Input: part model. Units: mm. Frame: model coordinates. A direction names the side the tool comes from. Coordinates: 2 decimals unless noted, no trailing zeros. Write each loop counter-clockwise with the first axis right and the second up, starting at its lowest first coordinate (ties: lowest second). Pieces come first, ordered by that corner, then holes. Notation, with made-up numbers: (7.5, 42.5) -> (56.5, 42.5) arc R25 cw to (56.5, 65.5) -> close; hole circle Ø9 at (-21, -36.75). An arc over 180 degrees is marked (long way). One line per question, with ' | ' between items. Start each with the question number.
```python
from build123d import *

# Parameters (mm, degrees)
SKETCH1_W           = 25.4
SKETCH1_H           = 24.3078
BOSS_EXTRUDE1_DEPTH = 1.016
SKETCH2_R           = 1.016
CUT_EXTRUDE1_DEPTH  = 10
SKETCH3_W           = 21.9964
SKETCH3_H           = 5.588
BOSS_EXTRUDE2_DEPTH = 2.413
BOSS_EXTRUDE3_DEPTH = 3.175
BOSS_EXTRUDE4_DEPTH = 3.81
SKETCH6_R           = 6.096408591
BOSS_EXTRUDE5_DEPTH = 4.572
SKETCH9_R           = 1.5621
BOSS_EXTRUDE6_DEPTH = 1.0668
FILLET1_R           = 0.25
SKETCH10_R          = 1
CUT_EXTRUDE2_DEPTH  = 1


with BuildPart() as part:
    # Sketch1 → Boss-Extrude1 (new body)
    with BuildSketch(Plane(origin=(0, 0, 0), x_dir=(1, 0, 0), z_dir=(0, 1, 0))):
        with Locations((4.969417476, -5.139336893)):
            Rectangle(SKETCH1_W, SKETCH1_H)
    extrude(amount=BOSS_EXTRUDE1_DEPTH)

    # Sketch2 → Cut-Extrude1 (cut)
    with BuildSketch(Plane(origin=(0, 1.016, 0), x_dir=(1, 0, 0), z_dir=(0, 1, 0))):
        with Locations((-5.596982524, 4.880963107)):
            Circle(SKETCH2_R)
        with Locations((-5.596982524, -8.504836893)):
            Circle(SKETCH2_R)
        with Locations((15.535817476, 4.880963107)):
            Circle(SKETCH2_R)
        with Locations((15.535817476, -8.504836893)):
            Circle(SKETCH2_R)
    extrude(amount=-CUT_EXTRUDE1_DEPTH, mode=Mode.SUBTRACT)

    # Sketch3 → Boss-Extrude2 (add)
    with BuildSketch(Plane(origin=(0, 1.016, 0), x_dir=(1, 0, 0), z_dir=(0, 1, 0))):
        with Locations((4.969417476, -13.991236893)):
            Rectangle(SKETCH3_W, SKETCH3_H)
    extrude(amount=BOSS_EXTRUDE2_DEPTH)

    # Sketch4 → Boss-Extrude3 (add)
    with BuildSketch(Plane(origin=(0, 1.016, 0), x_dir=(1, 0, 0), z_dir=(0, 1, 0))):
        with BuildLine():
            Line((-1.634582524, 5.109563107), (11.573417476, 5.109563107))
            Line((11.573417476, 5.109563107), (11.573417476, 0.499463107))
            Line((11.573417476, 0.499463107), (14.024517476, 0.499463107))
            ThreePointArc((14.024517476, 0.499463107), (16.018417476, -1.494436893), (14.024517476, -3.488336893))
            Line((14.024517476, -3.488336893), (11.573417476, -3.488336893))
            Line((11.573417476, -3.488336893), (11.573417476, -8.098436893))
            Line((11.573417476, -8.098436893), (-1.634582524, -8.098436893))
            Line((-1.634582524, -8.098436893), (-1.634582524, -3.488336893))
            Line((-1.634582524, -3.488336893), (-4.085682524, -3.488336893))
            ThreePointArc((-4.085682524, -3.488336893), (-6.079582524, -1.494436893), (-4.085682524, 0.499463107))
            Line((-4.085682524, 0.499463107), (-1.634582524, 0.499463107))
            Line((-1.634582524, 0.499463107), (-1.634582524, 5.109563107))
        make_face()
    extrude(amount=BOSS_EXTRUDE3_DEPTH)

    # Sketch5 → Boss-Extrude4 (add)
    with BuildSketch(Plane(origin=(0, 4.191, 0), x_dir=(1, 0, 0), z_dir=(0, 1, 0))):
        with BuildLine():
            Line((6.671833409, -8.098436893), (3.267001542, -8.098436893))
            ThreePointArc((3.267001542, -8.098436893), (-1.850482524, -1.494436893), (3.267001542, 5.109563107))
            Line((3.267001542, 5.109563107), (4.969417476, 5.109563107))
            Line((4.969417476, 5.109563107), (6.671833409, 5.109563107))
            ThreePointArc((6.671833409, 5.109563107), (11.789317476, -1.494436893), (6.671833409, -8.098436893))
        make_face()
    extrude(amount=BOSS_EXTRUDE4_DEPTH)

    # Sketch6 → Boss-Extrude5 (add)
    with BuildSketch(Plane(origin=(0, 8.001, 0), x_dir=(1, 0, 0), z_dir=(0, 1, 0))):
        with Locations((4.969417476, -1.494436893)):
            Circle(SKETCH6_R)
    extrude(amount=BOSS_EXTRUDE5_DEPTH)

    # Sketch8 → Revolve1 (revolve)
    with BuildSketch(Plane(origin=(4.969417476, 12.573, 1.494436893), x_dir=(0, 0, 1), z_dir=(-1, 0, 0))):
        with BuildLine():
            Line((-4.44130706, 5.035394986), (-6.985, 3.302))
            Line((-6.985, 3.302), (-6.985, 0))
            Line((-6.985, 0), (0, 0))
            Line((0, 0), (0, 6.35))
            add(Edge.make_bspline(
                [(0, 6.35), (-2.343173103, 6.35), (-3.129648943, 5.88240785), (-4.44130706, 5.035394986)],
                knots=[0, 0, 0, 0, 1, 1, 1, 1], degree=3))
        make_face()
    revolve(axis=Axis((4.969417476, 12.573, 1.494436893), (0, 1, 0)))

    # Sketch9 → Boss-Extrude6 (add)
    with BuildSketch(Plane.XZ):
        with Locations((14.430917476, 1.659536893)):
            Circle(SKETCH9_R)
        with Locations((-4.492082524, 1.659536893)):
            Circle(SKETCH9_R)
    extrude(amount=BOSS_EXTRUDE6_DEPTH)

    # Fillet1
    fillet1_edges = [part.edges().sort_by_distance(p)[0] for p in [
        (12.868817476, -1.0668, 1.659536893),
        (-6.054182524, -1.0668, 1.659536893),
    ]]
    fillet(fillet1_edges, radius=FILLET1_R)

    # Sketch10 → Cut-Extrude2 (cut)
    with BuildSketch(Plane.XZ):
        with Locations((4.969417476, 5.139336893)):
            Circle(SKETCH10_R)
    extrude(amount=-CUT_EXTRUDE2_DEPTH, mode=Mode.SUBTRACT)


solid = part.part
```
1) Section A-A, the plane z = 14. Return loops of the section in (x, y), then the cut area to 3 significant figures.
2) First-contact query: P1, Ø2, axis at x = 4, z = -4, coming from the -Y side; P2, Ø3.5, axis at y = 3, z = -3, coming from the -X side; P3, Ø2, axis at x = 5, y = 5, coming from the -Z side; P4, Ø3.5, axis at y = 2, z = 5, coming from the -X side. Flat tips, straight axial feed; report the tip coordinate or a pass-through.
3) Section C-C, the plane x = 15. Give the number of separate pieces and of enclosed holes in the cut face, then the cut area to 3 significant figures.
4) Ray query, line 1 (Y direction, x = -6, z = 0.5); line 2 (Y direction, x = 4.5, z = 11.5); line 3 (Z direction, x = 4.25, y = 7.5). Return the intervals inside material, ascending.
5) Section D-D, the plane y = 15. Return loops of the section in (x, z) (3 decimals).
6) Pull-direction query (X, two-part tool) for faces 4 (the face through (5.923, 0.493, 5.44)), 5 (the face through (-7.731, 0.5, 5.3)), 6 (the face through (5, 1, 5)), 7 (the face through (8, 8.001, 7)); classes: released by +X, released by -X, zero draft, split by the parting line, or undercut.
7) Section B-B, the plane y = 5.25. Return loops of the section in (x, z).
8) Access query for faces 1 (the face through (16.018, 2.581, 1.451)), 2 (the face through (15.968, 2, 14)), 3 (the face through (5, 3.429, 14)). Directions: +Z, -Z, +X, -X, +Y, -Y. A direction counts if a zero-diameter tool reaches every point of the face in a straight line with its end or side. Return the directions, or none.
Answer block:
1) outline: (-7.73, 0) -> (17.67, 0) -> (17.67, 1.02) -> (15.97, 1.02) -> (15.97, 3.43) -> (-6.03, 3.43) -> (-6.03, 1.02) -> (-7.73, 1.02) -> close | area: 78.9 mm2
2) P1: stops at y = 0 | P2: stops at x = -1.63 | P3: stops at z = -5.11 | P4: stops at x = -7.73
3) separate pieces: 3 | enclosed holes: 0 | area: 48.8 mm2
4) line 1: y = 0 to 1.02 | line 2: y = 0 to 3.43 | line 3: z = -5.11 to 8.1
5) outline: circle Ø13.97 at (4.969, 1.494)
6) face 4: undercut | face 5: released by -X | face 6: undercut | face 7: zero draft
7) outline: (3.27, -5.11) -> (6.67, -5.11) arc R6.82 ccw to (6.67, 8.1) -> (3.27, 8.1) arc R6.82 ccw to start
8) face 1: +X, +Y | face 2: +Z, +X, +Y | face 3: +Z, +X, -X, +Y
